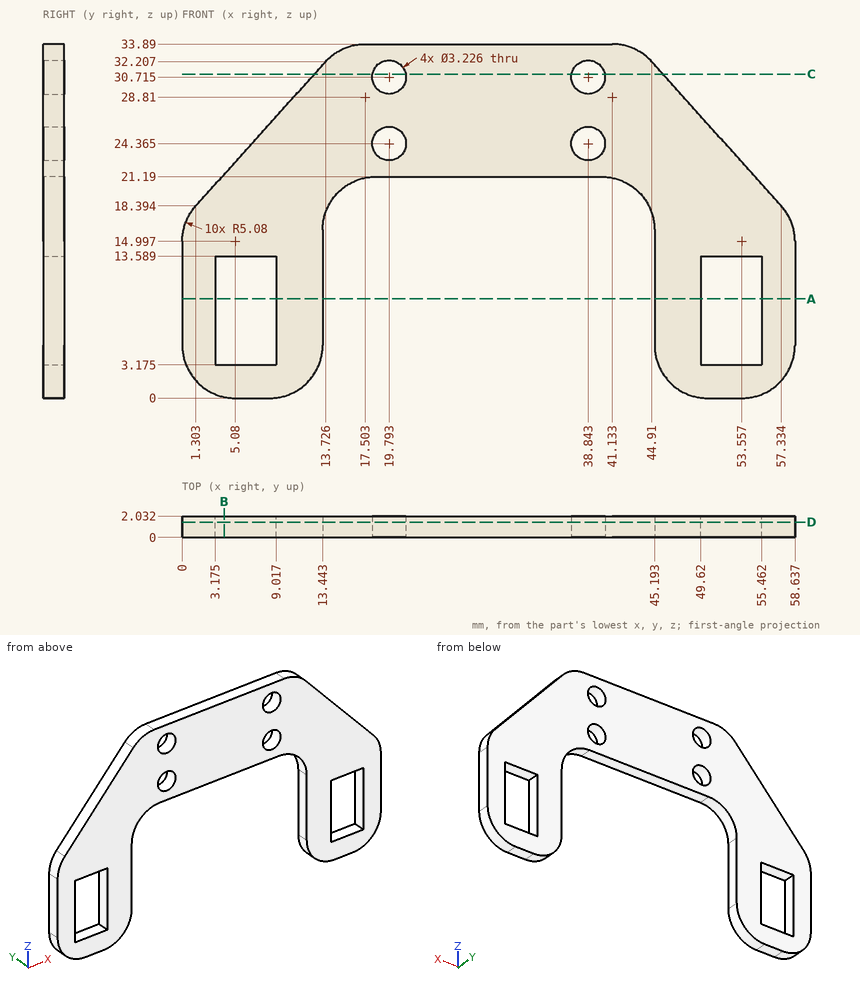
Input: dimensioned drawing with shaded views. Units: mm. Origin: part minimum x, y, z. Round coordinates to 2 decimals unless told otherwise and drop trailing zeros. Write each loop counter-clockwise with the first axis right and the second up, starting at its lowest first coordinate (ties: lowest second). Pieces come first, ordered by that corner, then holes. Notation, with made-up numbers: (66.25, 78.25) - (107.25, 78.25) arc R25 ccw to (107.25, 99.25) - close; hole circle Ø3 at (89, 17). An arc over 180 degrees is marked (long way). Write item = value, one per line.
(1) Material intervals for probe 1 along X at (y, z) = (0.4, 7) (1 decimal); probe 2 along Z at (x, y) = (39, 0.55); probe 3 along X at (y, z) = (1.6, 15), sorted ascending.
Geometry check:
probe_1 = 0 to 3.2, 9 to 13.4, 45.2 to 49.6, 55.5 to 58.6
probe_2 = 21.19 to 22.76, 25.97 to 29.11, 32.32 to 33.89
probe_3 = 0 to 13.44, 45.19 to 58.64
(2) Section query B-B on x = 4. Output: boundary loops of the cut face in (y, z) (1 decimal).
Geometry check:
outline = (0, 0.1) - (2, 0.1) - (2, 3.2) - (0, 3.2) - close; (0, 13.6) - (2, 13.6) - (2, 21.4) - (0, 21.4) - close
(3) Section query D-D on y = 1.45. State how many separate pieces and enclosed holes the cut face has.
Geometry check:
separate_pieces = 1
enclosed_holes = 6
(4) Contact query for flat-ended pins moving along their axis: pin 1 Ø1 at (y, z) = (1.5, 9) entering from -X; pin 2 Ø1 at (y, z) = (1.5, 29) entering from +X (1 decimal); pin 3 Ø1 at (x, y) = (52, 0.5) entering from +Z. Output: stop coordinate, or through.
Geometry check:
pin_1 = 0
pin_2 = 48.2
pin_3 = 24.88
(5) Section query A-A on z = 9.5. Output: boundary loops of the cut face in (x, y) (1 decimal).
Geometry check:
outline = (0, 0) - (3.2, 0) - (3.2, 2) - (0, 2) - close; (9, 0) - (13.4, 0) - (13.4, 2) - (9, 2) - close; (45.2, 0) - (49.6, 0) - (49.6, 2) - (45.2, 2) - close; (55.5, 0) - (58.6, 0) - (58.6, 2) - (55.5, 2) - close
(6) Section query C-C on z = 31. Output: boundary loops of the cut face in (x, y) (1 decimal).
Geometry check:
outline = (12.6, 0) - (18.2, 0) - (18.2, 2) - (12.6, 2) - close; (21.4, 0) - (37.3, 0) - (37.3, 2) - (21.4, 2) - close; (40.4, 0) - (46, 0) - (46, 2) - (40.4, 2) - close
